Design review of the part built by this model. Coordinates are the model's own, in mm. A direction names the side the tool comes from. Coordinates: 2 decimals unless noted, no trailing zeros. Write each loop counter-clockwise with the first axis right and the second up, starting at its lowest first coordinate (ties: lowest second). Pieces come first, ordered by that corner, then holes. Notation, with made-up numbers: (18.5, 59) - (74.5, 59) arc R13 cw to (74.5, 78) - close; hole circle Ø4 at (7.25, 78). An arc over 180 degrees is marked (long way). Use a Markdown table: item, result.
from build123d import *

# Parameters (mm, degrees)
SKETCH_R  = 1.85
PAD_DEPTH = 3


with BuildPart() as part:
    # Sketch → Pad (new body)
    with BuildSketch(Plane.XY):
        with BuildLine():
            ThreePointArc((-10, 0), (0, -10), (10, 0))
            Line((10, 0), (10, 59.547349))
            ThreePointArc((10, 59.547349), (12.484765, 68.50486), (3.193049, 68.778855))
            Line((-3.193049, 68.778855), (3.193049, 68.778855))
            ThreePointArc((-3.193049, 68.778855), (-12.484765, 68.50486), (-10, 59.547349))
            Line((-10, 59.547349), (-10, 0))
        make_face()
        with Locations((8, 65)):
            Circle(SKETCH_R, mode=Mode.SUBTRACT)
        with Locations((-8, 65)):
            Circle(SKETCH_R, mode=Mode.SUBTRACT)
        with BuildLine():
            ThreePointArc((4, 11), (0, 15), (-4, 11))
            Line((-4, 11), (-4, 4))
            ThreePointArc((-4, 4), (0, 0), (4, 4))
            Line((4, 4), (4, 11))
        make_face(mode=Mode.SUBTRACT)
    extrude(amount=PAD_DEPTH)


solid = part.part
(1) Take a section at B-B on x = 0. Write out the cut boundary in (y, z), and give its area (3 significant figures).
Determined:
| item | result |
|---|---|
| outline | (-10, 0) - (0, 0) - (0, 3) - (-10, 3) - close; (15, 0) - (68.78, 0) - (68.78, 3) - (15, 3) - close |
| area | 191 mm2 |
(2) Draft analysis for pull direction X (two halves, no side actions). For faces 4 (the cylindrical face through (-12.394, 68.624, 1.479)), 5 (the cylindrical face through (0, -10, 1)), 6 (the flat face through (0, 40, 0)), state which applies: +X half, -X half, draft (parallel to the pull), parting line (faces both ways), or undercut.
Determined:
| item | result |
|---|---|
| face 4 | undercut |
| face 5 | parting line |
| face 6 | draft |
(3) Take a section at C-C on z = 1.15. Write out the cut boundary in (x, y).
Determined:
| item | result |
|---|---|
| outline | (-10, 0) arc R10 ccw to (10, 0) - (10, 59.55) arc R5.91 ccw (long way) to (3.19, 68.78) - (-3.19, 68.78) arc R5.91 ccw (long way) to (-10, 59.55) - close; hole circle Ø3.7 at (-8, 65); hole (-4, 4) arc R4 ccw to (4, 4) - (4, 11) arc R4 ccw to (-4, 11) - close; hole circle Ø3.7 at (8, 65) |
(4) Machinability: for faces 1 (the flat face through (0, 68.779, 1)), 2 (the cylindrical face through (0, 15, 1)), 3 (the flat face through (-10, 30, 1)), which of the approach directions +Z, -Z, +X, -X, +Y, -Y give a long, thin tool a straight path to every point of the face, cutting with its end or side? Answer none if there is none.
Determined:
| item | result |
|---|---|
| face 1 | +Z, -Z, +Y |
| face 2 | +Z, -Z |
| face 3 | +Z, -Z, -X, -Y |
(5) Take a section at A-A on y = 65. Write out the cut boundary in (x, z).
Determined:
| item | result |
|---|---|
| outline | (-13.64, 0) - (-9.85, 0) - (-9.85, 3) - (-13.64, 3) - close; (-6.15, 0) - (6.15, 0) - (6.15, 3) - (-6.15, 3) - close; (9.85, 0) - (13.64, 0) - (13.64, 3) - (9.85, 3) - close |
(6) For pin 1 (3 mm diameter, centred on x = 3, y = 11.5, fed in from -Z); pin 2 (1.5 mm diameter, centred on y = 35.5, z = 1, fed in from -X); pin 3 (3.5 mm diameter, centred on x = 8, y = 65, fed in from +Z); pin 4 (1.5 mm diameter, centred on y = 7.5, z = 1.5, fed in from +X), all flat-tipped, find the tip position at first contact; note any pin that passes through.
Determined:
| item | result |
|---|---|
| pin 1 | z = 0 |
| pin 2 | x = -10 |
| pin 3 | through |
| pin 4 | x = 10 |
(7) Take a section at D-D on x = -8. Write out the cut boundary in (y, z).
Determined:
| item | result |
|---|---|
| outline | (-6, 0) - (63.15, 0) - (63.15, 3) - (-6, 3) - close; (66.85, 0) - (70.9, 0) - (70.9, 3) - (66.85, 3) - close |
(8) For L1, parallel to X at y = 65, z = 1.15; L2, parallel to X at y = 40, z = 1.35; L3, parallel to X at y = 2, z = 2.75, list the stretches that pass through material, from the lowest coordinate up. Write a range as from..to.
Determined:
| item | result |
|---|---|
| L1 | -13.64..-9.85, -6.15..6.15, 9.85..13.64 |
| L2 | -10..10 |
| L3 | -10..-3.46, 3.46..10 |
